Input: part model. Units: mm. Frame: model coordinates. Give positions to 0.01 mm unless a question says otherwise; leave off trailing zeros. Order: outer loops, then holes, each group sorted by start corner. A loop starts at its lowest first (then second) coordinate and runs counter-clockwise, first axis right, second up. Notation, with made-up numbers: (43.5, 43.5) -> (87.5, 43.5) arc R21 ccw to (87.5, 70.5) -> close; hole circle Ø11 at (76.5, 32). An arc over 180 degrees is marked (long way). Use a Markdown table: item, result. Add a question column.
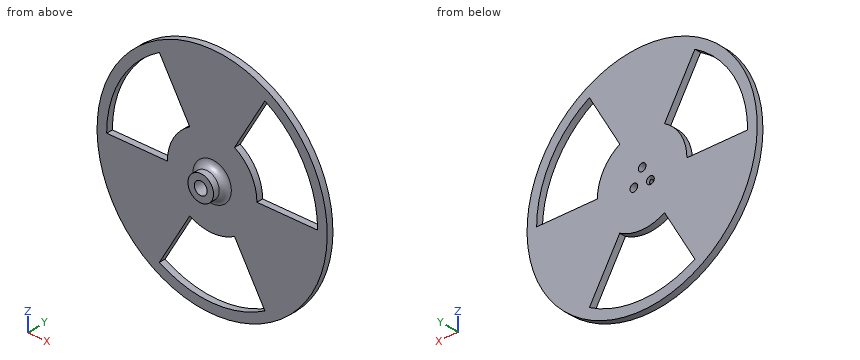
from build123d import *

# Parameters (mm, degrees)
SKETCH1_R           = 18
BOSS_EXTRUDE1_DEPTH = 1
SKETCH2_R           = 2
BOSS_EXTRUDE2_DEPTH = 2
SKETCH3_R           = 1
CUT_EXTRUDE1_DEPTH  = 2.5
FILLET1_R           = 1
SKETCH4_R           = 0.6
CUT_EXTRUDE2_DEPTH  = 1


with BuildPart() as part:
    # Sketch1 → Boss-Extrude1 (new body)
    with BuildSketch(Plane(origin=(0, 0, 0), x_dir=(1, 0, 0), z_dir=(0, 1, 0))):
        with Locations(Location((0, 0, 0), (0, 0, 270))):
            Circle(SKETCH1_R)
    extrude(amount=BOSS_EXTRUDE1_DEPTH)

    # Sketch2 → Boss-Extrude2 (add)
    with BuildSketch(Plane.XZ):
        with Locations(Location((0, 0, 0), (0, 0, 90))):
            Circle(SKETCH2_R)
    extrude(amount=BOSS_EXTRUDE2_DEPTH)

    # Sketch3 → Cut-Extrude1 (cut)
    with BuildSketch(Plane.XZ.offset(2)):
        with Locations(Location((0, 0, 0), (0, 0, 270))):
            Circle(SKETCH3_R)
    extrude(amount=-CUT_EXTRUDE1_DEPTH, mode=Mode.SUBTRACT)

    # Fillet1
    fillet1_edges = [part.edges().sort_by_distance(p)[0] for p in [
        (0, 0, -2),
    ]]
    fillet(fillet1_edges, radius=FILLET1_R)

    # Sketch4 → Cut-Extrude2 (cut)
    with BuildSketch(Plane(origin=(0, 1, 0), x_dir=(1, 0, 0), z_dir=(0, 1, 0))):
        with Locations(Location((1.299038106, 0.75, 0), (0, 0, 270))):
            Circle(SKETCH4_R)
        with Locations(Location((0, -1.5, 0), (0, 0, 270))):
            Circle(SKETCH4_R)
        with Locations(Location((-1.299038106, 0.75, 0), (0, 0, 270))):
            Circle(SKETCH4_R)
        with BuildLine():
            Line((-3.5, 6.062177826), (-8.25, 14.289419162))
            ThreePointArc((-8.25, 14.289419162), (0, 16.5), (8.25, 14.289419162))
            Line((8.25, 14.289419162), (3.5, 6.062177826))
            ThreePointArc((3.5, 6.062177826), (0, 7), (-3.5, 6.062177826))
        make_face()
        with BuildLine():
            Line((7, 0), (16.5, 0))
            ThreePointArc((16.5, 0), (14.289419162, -8.25), (8.25, -14.289419162))
            Line((8.25, -14.289419162), (3.5, -6.062177826))
            ThreePointArc((3.5, -6.062177826), (6.062177826, -3.5), (7, 0))
        make_face()
        with BuildLine():
            Line((-3.5, -6.062177826), (-8.25, -14.289419162))
            ThreePointArc((-8.25, -14.289419162), (-14.289419162, -8.25), (-16.5, 0))
            Line((-16.5, 0), (-7, 0))
            ThreePointArc((-7, 0), (-6.062177826, -3.5), (-3.5, -6.062177826))
        make_face()
    extrude(amount=-CUT_EXTRUDE2_DEPTH, mode=Mode.SUBTRACT)


solid = part.part
Q1. First-contact query: pin 1 (1.1 mm diameter, centred on x = -12.5, y = 0.5, fed in from +Z); pin 2 (1 mm diameter, centred on x = -9, y = 0, fed in from -Z); pin 3 (2 mm diameter, centred on x = -12.5, z = -12, fed in from -Y); pin 4 (1 mm diameter, centred on x = 6.5, y = -1, fed in from +Z). Flat tips, straight axial feed; report the tip coordinate or a pass-through.
Q2. Section query A-A (x = -11). Return loops of the section in (y, z), plus the area to 3 significant figures.
Q3. Section query D-D (z = 15). Return loops of the section in (x, y), plus the area to 3 significant figures.
Q4. Ray query, line 1 (X direction, y = 0.7, z = -0.75); line 2 (X direction, y = 0.65, z = 8); line 3 (X direction, y = 0.6, z = 1.5). Return the intervals inside material, ascending.
Q5. Section query C-C (z = 8.5). Return loops of the section in (x, y), plus the area to 3 significant figures.
Q6. Section query B-B (z = -10.5). Return loops of the section in (x, y), plus the area to 3 significant figures.
Solution:
| question | item | result |
|---|---|---|
| 1 | pin 1 | stops at z = 13.46 |
| 1 | pin 2 | stops at z = -15.87 |
| 1 | pin 3 | stops at y = 0 |
| 1 | pin 4 | passes through |
| 2 | outline | (0, -14.25) -> (1, -14.25) -> (1, 0) -> (0, 0) -> close; (0, 12.3) -> (1, 12.3) -> (1, 14.25) -> (0, 14.25) -> close |
| 2 | area | 16.2 mm² |
| 3 | outline | (-9.95, 0) -> (9.95, 0) -> (9.95, 1) -> (-9.95, 1) -> close |
| 3 | area | 19.9 mm² |
| 4 | line 1 | x = -17.98 to -1.9, -0.7 to 0.7, 1.9 to 17.98 |
| 4 | line 2 | x = -16.12 to -14.43, -4.62 to 4.62, 14.43 to 16.12 |
| 4 | line 3 | x = -17.94 to -16.43, -6.84 to -0.6, 0.6 to 6.84, 16.43 to 17.94 |
| 5 | outline | (-15.87, 0) -> (-14.14, 0) -> (-14.14, 1) -> (-15.87, 1) -> close; (-4.91, 0) -> (4.91, 0) -> (4.91, 1) -> (-4.91, 1) -> close; (14.14, 0) -> (15.87, 0) -> (15.87, 1) -> (14.14, 1) -> close |
| 5 | area | 13.3 mm² |
| 6 | outline | (-14.62, 0) -> (-6.06, 0) -> (-6.06, 1) -> (-14.62, 1) -> close; (6.06, 0) -> (14.62, 0) -> (14.62, 1) -> (6.06, 1) -> close |
| 6 | area | 17.1 mm² |
